Print and shaded views of the part. All mm, measured from the part's lowest x, y and z. A direction names the side the tool comes from. Coordinates: 2 decimals unless noted, no trailing zeros. Loops run counter-clockwise (first coordinate to the right, second up) from the corner with the lowest first, then second, coordinate; pieces in that order, holes last. Notation, with made-up numbers: M 40.25,-36.75 L 57.25,-36.75 A22 ccw 57.25,-23.75 Z; hole C 34.25,20.5 d8. An arc over 180 degrees is marked long. Use a Markdown table: item, result. Add a question column.
1) Pin check, flat tips, straight feed: pin 1 Ø4 at (x, y) = (10.5, 6) entering from -Z; pin 2 Ø1 at (x, z) = (5.5, 10) entering from -Y; pin 3 Ø4 at (y, z) = (3.5, 3.5) entering from +X. Stop position of each tip, or through.
2) Tool access for the marked faces 1 and 2: list every direction of +Z, -Z, +X, -X, +Y, -Y with a clear straight run to the whole face (end or side of a thin tool).
3) Band-saw the part on C-C (z = 2.25). List the corners of the cut face in (x, y), plus the area to 3 significant figures.
4) Wall check: probe 1 along Z at (x, y) = (1.5, 5.25); probe 2 along X at (y, z) = (8.5, 7); probe 3 along X at (y, z) = (13, 2). Give the ranges that are in metal, low to high. Write a range as from..to.
5) Band-saw the part on A-A (x = 7.5). List the corners of the cut face in (y, z), plus the area to 3 significant figures.
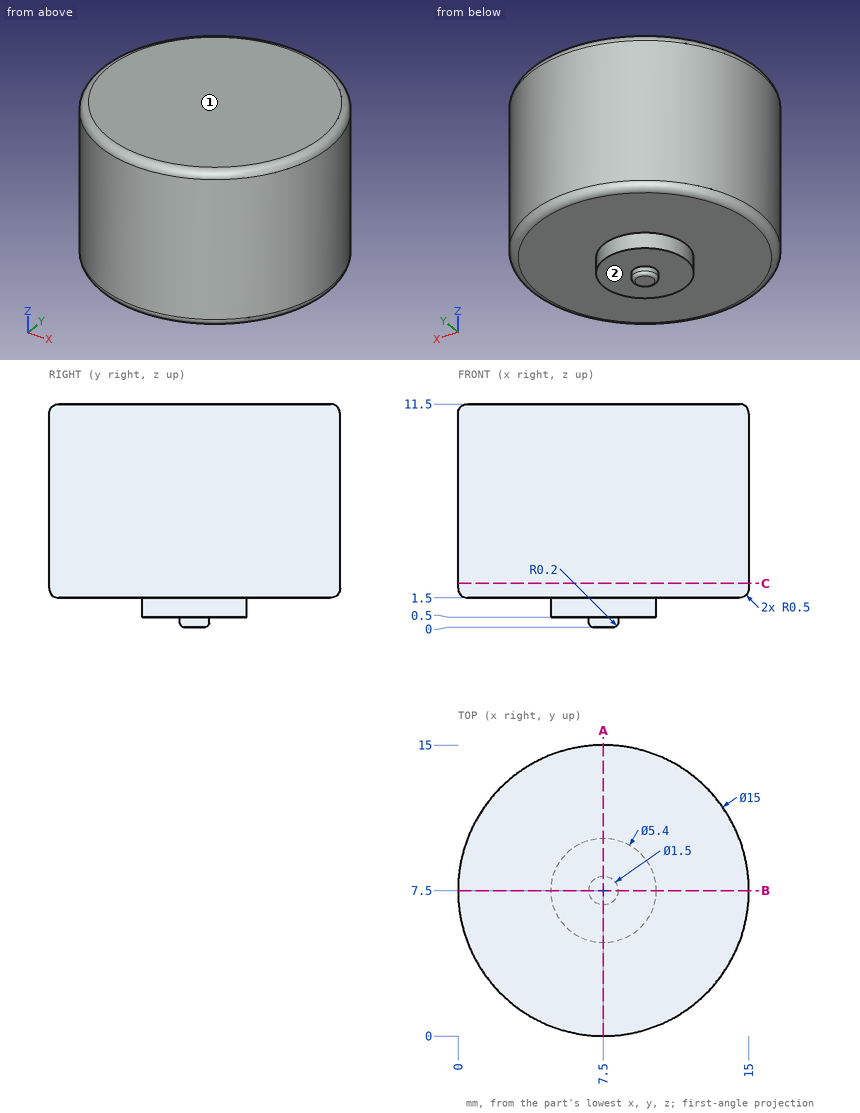
Entries:
| question | item | result |
|---|---|---|
| 1 | pin 1 | z = 0.5 |
| 1 | pin 2 | y = 0.15 |
| 1 | pin 3 | x = 14.73 |
| 2 | face 1 | +Z, +X, -X, +Y, -Y |
| 2 | face 2 | -Z |
| 3 | outline | C 7.5,7.5 d15 |
| 3 | area | 177 mm2 |
| 4 | probe 1 | 1.5..11.5 |
| 4 | probe 2 | 0.07..14.93 |
| 4 | probe 3 | 2.4..12.6 |
| 5 | outline | M 0,2 A0.5 ccw 0.5,1.5 L 4.8,1.5 L 4.8,0.5 L 6.75,0.5 L 6.75,0.2 A0.2 ccw 6.95,0 L 8.05,0 A0.2 ccw 8.25,0.2 L 8.25,0.5 L 10.2,0.5 L 10.2,1.5 L 14.5,1.5 A0.5 ccw 15,2 L 15,11 A0.5 ccw 14.5,11.5 L 0.5,11.5 A0.5 ccw 0,11 Z |
| 5 | area | 156 mm2 |
